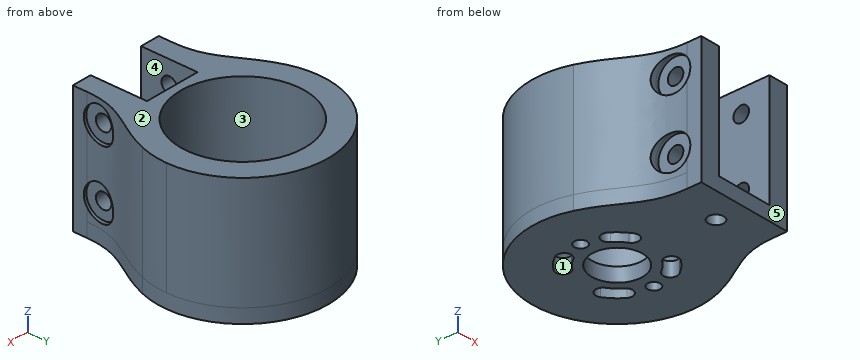
```python
from build123d import *
from build123d.topology import SkipClean

# Parameters (mm, degrees)
SKETCH1_R                              = 22
BOSS_EXTRUDE1_DEPTH                    = 40
CBORE_FOR_M5_HEX_HEAD_BOLT1_AT_2_COUNT = 2
CBORE_FOR_M5_HEX_HEAD_BOLT1_AT_2_PITCH = 24
CUT_EXTRUDE1_DEPTH                     = 90.923150822
BOSS_EXTRUDE2_START                    = 5
SKETCH6_R                              = 9
BOSS_EXTRUDE2_DEPTH                    = 5
M5_CLEARANCE_HOLE1_D                   = 5.5
M5_CLEARANCE_HOLE1_DEPTH               = 12
M5_CLEARANCE_HOLE1_TIP                 = 1.652366702
M4_CLEARANCE_HOLE1_D                   = 4.5
M4_CLEARANCE_HOLE1_DEPTH               = 12
M4_CLEARANCE_HOLE1_TIP                 = 1.351936393
CUT_EXTRUDE2_START                     = -5
SKETCH11_R                             = 2.25
CUT_EXTRUDE2_DEPTH                     = 5


with BuildPart() as part:
    # Sketch1 → Boss-Extrude1 (new body)
    # profile 1 of 7: a face of its own
    with BuildSketch(Plane.XY):
        with BuildLine():
            Line((-17, 10), (-10, 10))
            Line((-10, 10), (10, 10))
            Line((10, 10), (17, 10))
            ThreePointArc((17, 10), (23.968955432, 16.574767966), (28.530685235, 25))
            ThreePointArc((28.530685235, 25), (29.803959698, 29.928118072), (30.232432916, 35))
            ThreePointArc((30.232432916, 35), (-5.071881928, 64.803959698), (-28.530685235, 25))
            ThreePointArc((-28.530685235, 25), (-23.968955432, 16.574767966), (-17, 10))
        make_face()
        with Locations((0, 35)):
            Circle(SKETCH1_R, mode=Mode.SUBTRACT)
    # profile 2 of 7: a face of its own
    with BuildSketch(Plane.XY):
        with BuildLine():
            Line((-17, -5), (-17, 10))
            ThreePointArc((-17, 10), (-23.968955432, 16.574767966), (-28.530685235, 25))
            add(Edge.make_bspline(
                [(-28.530685235, 25), (-24.136929726, 12.464314457), (-17, 8.619402075), (-17, -5)],
                knots=[0, 0, 0, 0, 1, 1, 1, 1], degree=3))
        make_face()
    # profile 3 of 7: a face of its own
    with BuildSketch(Plane.XY):
        with BuildLine():
            Line((-17, -10), (-10, -10))
            Line((-10, -10), (-10, 6.469314765))
            ThreePointArc((-10, 6.469314765), (-13.614934247, 8.006786678), (-17, 10))
            Line((-17, 10), (-17, -5))
            Line((-17, -5), (-17, -10))
        make_face()
    # profile 4 of 7: a face of its own
    with BuildSketch(Plane.XY):
        with BuildLine():
            Line((10, 6.469314765), (10, -10))
            Line((10, -10), (17, -10))
            Line((17, -10), (17, -5))
            Line((17, -5), (17, 10))
            ThreePointArc((17, 10), (13.614934247, 8.006786678), (10, 6.469314765))
        make_face()
    # profile 5 of 7: a face of its own
    with BuildSketch(Plane.XY):
        with BuildLine():
            ThreePointArc((28.530685235, 25), (23.968955432, 16.574767966), (17, 10))
            Line((17, 10), (17, -5))
            add(Edge.make_bspline(
                [(28.530685235, 25), (24.136929726, 12.464314457), (17, 8.619402075), (17, -5)],
                knots=[0, 0, 0, 0, 1, 1, 1, 1], degree=3))
        make_face()
    # profile 6 of 7: a face of its own
    with BuildSketch(Plane.XY):
        with BuildLine():
            ThreePointArc((-17, 10), (-13.614934247, 8.006786678), (-10, 6.469314765))
            Line((-10, 6.469314765), (-10, 10))
            Line((-10, 10), (-17, 10))
        make_face()
    # profile 7 of 7: a face of its own
    with BuildSketch(Plane.XY):
        with BuildLine():
            Line((10, 10), (10, 6.469314765))
            ThreePointArc((10, 6.469314765), (13.614934247, 8.006786678), (17, 10))
            Line((17, 10), (10, 10))
        make_face()
    extrude(amount=BOSS_EXTRUDE1_DEPTH)

    # Sketch4 → CBORE for M5 Hex Head Bolt1 (revolve, cut)
    with BuildSketch(Plane(origin=(-17, 0, 8), x_dir=(0, 0, 1), z_dir=(0, 1, 0))):
        Polygon((0, 0), (0, 13.652366702), (2.75, 12), (2.75, 1), (6.12, 1), (6.12, 0), align=None)
    cbore_for_m5_hex_head_bolt1 = revolve(axis=Axis((-23.35, 0, 8), (1, 0, 0)), mode=Mode.SUBTRACT)

    # CBORE for M5 Hex Head Bolt1 at 2: CBORE for M5 Hex Head Bolt1 ×2
    with Locations(*[(0, 0, i * CBORE_FOR_M5_HEX_HEAD_BOLT1_AT_2_PITCH) for i in range(1, CBORE_FOR_M5_HEX_HEAD_BOLT1_AT_2_COUNT)]):
        add(cbore_for_m5_hex_head_bolt1, mode=Mode.SUBTRACT)

    # Sketch5 → Cut-Extrude1 (cut, through all)
    with BuildSketch(Plane.ZY.offset(17)):
        with BuildLine():
            ThreePointArc((14.12, 0), (5.184290916, 5.433799992), (4.4709208, -5))
            ThreePointArc((4.4709208, -5), (8, -6.12), (11.5290792, -5))
            ThreePointArc((11.5290792, -5), (13.433799992, -2.815709084), (14.12, 0))
        make_face()
        with BuildLine():
            ThreePointArc((38.12, 0), (29.184290916, 5.433799992), (28.4709208, -5))
            ThreePointArc((28.4709208, -5), (32, -6.12), (35.5290792, -5))
            ThreePointArc((35.5290792, -5), (37.433799992, -2.815709084), (38.12, 0))
        make_face()
    cut_extrude1 = extrude(amount=CUT_EXTRUDE1_DEPTH, mode=Mode.SUBTRACT)

    # Mirror1: CBORE for M5 Hex Head Bolt1, Cut-Extrude1 across plane
    add(cbore_for_m5_hex_head_bolt1.mirror(Plane(origin=(0, 0, 0), x_dir=(0, 0, 1), z_dir=(1, 0, 0))), mode=Mode.SUBTRACT)
    add(cut_extrude1.mirror(Plane(origin=(0, 0, 0), x_dir=(0, 0, 1), z_dir=(1, 0, 0))), mode=Mode.SUBTRACT)

    # Mirror1 copy 1 sketch → Mirror1 copy 1 (revolve, cut)
    with BuildSketch(Plane(origin=(17, 0, 32), x_dir=(0, 0, 1), z_dir=(0, 1, 0))):
        Polygon((0, 0), (0, -13.652366702), (2.75, -12), (2.75, -1), (6.12, -1), (6.12, 0), align=None)
    revolve(axis=Axis((23.35, 0, 32), (1, 0, 0)), mode=Mode.SUBTRACT)

    # Sketch6 → Boss-Extrude2 (add)
    with SkipClean():  # the faces are left unmerged after this step: merging them gives an invalid solid
        with BuildSketch(Plane(origin=(0, 0, 0), x_dir=(-1, 0, 0), z_dir=(0, 0, -1)).offset(BOSS_EXTRUDE2_START)):
            with BuildLine():
                Line((17, -10), (17, -5))
                add(Edge.make_bspline(
                    [(28.530685235, 25), (24.136929726, 12.464314457), (17, 8.619402075), (17, -5)],
                    knots=[0, 0, 0, 0, 1, 1, 1, 1], degree=3))
                ThreePointArc((28.530685235, 25), (0, 65.232432916), (-28.530685235, 25))
                add(Edge.make_bspline(
                    [(-28.530685235, 25), (-24.136929726, 12.464314457), (-17, 8.619402075), (-17, -5)],
                    knots=[0, 0, 0, 0, 1, 1, 1, 1], degree=3))
                Line((-17, -5), (-17, -10))
                Line((-17, -10), (17, -10))
            make_face()
            with Locations((0, 35)):
                Circle(SKETCH6_R, mode=Mode.SUBTRACT)
        extrude(amount=-BOSS_EXTRUDE2_DEPTH)

    # M5 Clearance Hole1
    with Locations(Plane.XY):
        with Locations((0, 0)):
            Hole(M5_CLEARANCE_HOLE1_D / 2, depth=M5_CLEARANCE_HOLE1_DEPTH)
            with Locations((0, 0, -(M5_CLEARANCE_HOLE1_DEPTH + M5_CLEARANCE_HOLE1_TIP / 2))):  # 118° drill point
                Cone(0, M5_CLEARANCE_HOLE1_D / 2, M5_CLEARANCE_HOLE1_TIP, mode=Mode.SUBTRACT)

    # M4 Clearance Hole1
    with Locations(Plane(origin=(0, 0, -5), x_dir=(-1, 0, 0), z_dir=(0, 0, -1))):
        with Locations((-14.5, 35), (14.5, 35), (0, 35)):
            Hole(M4_CLEARANCE_HOLE1_D / 2, depth=M4_CLEARANCE_HOLE1_DEPTH)
            with Locations((0, 0, -(M4_CLEARANCE_HOLE1_DEPTH + M4_CLEARANCE_HOLE1_TIP / 2))):  # 118° drill point
                Cone(0, M4_CLEARANCE_HOLE1_D / 2, M4_CLEARANCE_HOLE1_TIP, mode=Mode.SUBTRACT)

    # Sketch11 → Cut-Extrude2 (cut)
    with SkipClean():  # the faces are left unmerged after this step: merging them gives an invalid solid
        with BuildSketch(Plane(origin=(0, 0, -5), x_dir=(-1, 0, 0), z_dir=(0, 0, -1)).offset(CUT_EXTRUDE2_START)):
            with Locations((-14.5, 35)):
                Circle(SKETCH11_R)
            with BuildLine():
                ThreePointArc((-9.287155609, 49.238986646), (-12.02081528, 47.02081528), (-14.238986646, 44.287155609))
                ThreePointArc((-14.238986646, 44.287155609), (-13.510776199, 40.827428807), (-10.051049397, 41.555639253))
                ThreePointArc((-10.051049397, 41.555639253), (-8.485281374, 43.485281374), (-6.555639253, 45.051049397))
                ThreePointArc((-6.555639253, 45.051049397), (-5.827428807, 48.510776199), (-9.287155609, 49.238986646))
            make_face()
            with BuildLine():
                ThreePointArc((10.051049397, 41.555639253), (8.485281374, 43.485281374), (6.555639253, 45.051049397))
                ThreePointArc((6.555639253, 45.051049397), (5.827428807, 48.510776199), (9.287155609, 49.238986646))
                ThreePointArc((9.287155609, 49.238986646), (12.02081528, 47.02081528), (14.238986646, 44.287155609))
                ThreePointArc((14.238986646, 44.287155609), (13.510776199, 40.827428807), (10.051049397, 41.555639253))
            make_face()
            with BuildLine():
                ThreePointArc((6.555639253, 24.948950603), (8.485281374, 26.514718626), (10.051049397, 28.444360747))
                ThreePointArc((10.051049397, 28.444360747), (13.510776199, 29.172571193), (14.238986646, 25.712844391))
                ThreePointArc((14.238986646, 25.712844391), (12.02081528, 22.97918472), (9.287155609, 20.761013354))
                ThreePointArc((9.287155609, 20.761013354), (5.827428807, 21.489223801), (6.555639253, 24.948950603))
            make_face()
            with BuildLine():
                ThreePointArc((-10.051049397, 28.444360747), (-8.485281374, 26.514718626), (-6.555639253, 24.948950603))
                ThreePointArc((-6.555639253, 24.948950603), (-5.827428807, 21.489223801), (-9.287155609, 20.761013354))
                ThreePointArc((-9.287155609, 20.761013354), (-12.02081528, 22.97918472), (-14.238986646, 25.712844391))
                ThreePointArc((-14.238986646, 25.712844391), (-13.510776199, 29.172571193), (-10.051049397, 28.444360747))
            make_face()
        extrude(amount=CUT_EXTRUDE2_DEPTH, mode=Mode.SUBTRACT)


solid = part.part
```
Here's how the part is built. I have some questions about the finished solid (model axes, mm). Face numbers are marked on the shaded views. A direction names the side the tool comes from. Round coordinates to 2 decimals unless told otherwise and drop trailing zeros. Write each loop counter-clockwise with the first axis right and the second up, starting at its lowest first coordinate (ties: lowest second). Pieces come first, ordered by that corner, then holes.
Q1. Which directions (+Z, -Z, +X, -X, +Y, -Y) give clear straight access to the entire face, cutting with the end or side of a thin tool? Please do the marked faces 3, 4 and 5.
Q2. If we section it at A-A on x = 0: Write out the boundary of the cut face in (y, z), plus the area to 3 significant figures.
Q3. If we mould it in two halves opening along X, with no side actions, what happens to the marked faces 1 and 2? For each: +X half, -X half, draft (parallel to the pull), parting line (faces both ways), or undercut.
Q4. Will these pins go through, and if not, where does the flat tip stop? P1, Ø13, axis at x = 3, y = 39.5, coming from the +Z side; P2, Ø7.5, axis at y = 0, z = 32, coming from the -X side; P3, Ø3, axis at y = 15.5, z = 25, coming from the +X side; P4, Ø3.5, axis at y = 0, z = 32, coming from the +X side.
Q5. If we section it at B-B on z = 32: Give the number of separate pieces and of enclosed holes in the cut face, plus the area to 3 significant figures.
Q6. Please list where these lines run through material, in increasing order: probe 1 along Z at (x, y) = (16.25, 0); probe 2 along Y at (x, z) = (-12, 8); probe 3 along Y at (x, z) = (-13, 32).
Answer below:
1. face 3: +Z
1. face 4: +Z, -Y
1. face 5: +Z, -Z, +X, -X, -Y
2. outline: (-10, -5) - (-2.75, -5) - (-2.75, 0) - (-10, 0) - close; (2.75, -5) - (26, -5) - (26, 0) - (13, 0) - (13, 40) - (10, 40) - (10, 0) - (2.75, 0) - close; (44, -5) - (65.23, -5) - (65.23, 40) - (57, 40) - (57, 0) - (44, 0) - close
2. area: 708 mm2
3. face 1: undercut
3. face 2: draft
4. P1: stops at z = 0
4. P2: stops at x = -16
4. P3: stops at x = 24.91
4. P4: passes through
5. separate pieces: 3
5. enclosed holes: 1
5. area: 1,470 mm2
6. probe 1: z = -5 to 1.88, 14.12 to 25.88, 38.12 to 40
6. probe 2: y = -10 to -2.75, 2.75 to 16.56, 53.44 to 62.75
6. probe 3: y = -10 to -2.75, 2.75 to 17.25, 52.75 to 62.29
